Design review of the part built by this model. Coordinates are the model's own, in mm. A direction names the side the tool comes from. Give positions to 0.01 mm unless a question says otherwise; leave off trailing zeros. Order: outer loops, then holes, each group sorted by start corner. A loop starts at its lowest first (then second) coordinate and runs counter-clockwise, first axis right, second up. Notation, with made-up numbers: (36.25, 20) -> (45.25, 20) arc R20 ccw to (45.25, 30) -> close; hole circle Ø2 at (25, 15). An arc over 180 degrees is marked (long way). Return JSON: item names as keys, results as strings.
```python
from build123d import *

# Parameters (mm, degrees)
SKETCH1_R                                            = 60
SKETCH1_R_2                                          = 45
SKETCH1_R_3                                          = 40
BOSS_EXTRUDE3_DEPTH                                  = 10
SKETCH4_R                                            = 60
SKETCH4_R_2                                          = 50
BOSS_EXTRUDE4_DEPTH                                  = 6
SKETCH5_R                                            = 45
SKETCH5_R_2                                          = 42.5
BOSS_EXTRUDE5_DEPTH                                  = 8
FILLET1_R                                            = 2
SKETCH6_R                                            = 52.5
SKETCH6_R_2                                          = 42.5
CUT_EXTRUDE2_DEPTH                                   = 2
BOSS_EXTRUDE6_DEPTH                                  = 30
BOSS_EXTRUDE7_REACH                                  = 311.38
SKETCH8_R                                            = 20.5
SKETCH9_R                                            = 15
BOSS_EXTRUDE8_DEPTH                                  = 20
CUT_EXTRUDE3_DEPTH                                   = 250.99199991
CBORE_FOR_M3_HEXAGON_HEAD_BOLTS_FULL_THR_D           = 3.4
CBORE_FOR_M3_HEXAGON_HEAD_BOLTS_FULL_THR_CBORE_D     = 7
CBORE_FOR_M3_HEXAGON_HEAD_BOLTS_FULL_THR_CBORE_DEPTH = 2
CBORE_FOR_M3_HEXAGON_HEAD_BOLTS_FULL_2_D             = 3.4
CBORE_FOR_M3_HEXAGON_HEAD_BOLTS_FULL_2_CBORE_D       = 7
CBORE_FOR_M3_HEXAGON_HEAD_BOLTS_FULL_2_CBORE_DEPTH   = 2
SKETCH17_R                                           = 2.05
CUT_EXTRUDE4_DEPTH                                   = 15
SKETCH18_R                                           = 2.05
CUT_EXTRUDE5_DEPTH                                   = 15
SKETCH19_R                                           = 6
CUT_EXTRUDE6_DEPTH                                   = 2.5
SKETCH20_R                                           = 6
CUT_EXTRUDE7_DEPTH                                   = 2.5


with BuildPart() as part:
    # Sketch1 → Boss-Extrude3 (new body)
    # profile 1 of 3: a face of its own
    with BuildSketch(Plane(origin=(0, 0, 0), x_dir=(0, 0, -1), z_dir=(1, 0, 0))):
        Circle(SKETCH1_R)
        Circle(SKETCH1_R_2, mode=Mode.SUBTRACT)
    # profile 2 of 3: a face of its own
    with BuildSketch(Plane(origin=(0, 0, 0), x_dir=(0, 0, -1), z_dir=(1, 0, 0))):
        with BuildLine():
            ThreePointArc((-23.076923077, 55.384615385), (-60.776772972, 43.883864862), (-100, 40))
            Line((-100, 40), (-200, 40))
            ThreePointArc((-200, 40), (-171.715728753, 28.284271247), (-160, 0))
            ThreePointArc((-160, 0), (-171.715728753, -28.284271247), (-200, -40))
            Line((-200, -40), (-100, -40))
            ThreePointArc((-100, -40), (-60.776772972, -43.883864862), (-23.076923077, -55.384615385))
            ThreePointArc((-23.076923077, -55.384615385), (-60, 0), (-23.076923077, 55.384615385))
        make_face()
    # profile 3 of 3: a face of its own
    with BuildSketch(Plane(origin=(0, 0, 0), x_dir=(0, 0, -1), z_dir=(1, 0, 0))):
        with Locations((-200, 0)):
            Circle(SKETCH1_R_3)
    extrude(amount=BOSS_EXTRUDE3_DEPTH)

    # Sketch4 → Boss-Extrude4 (add)
    with BuildSketch(Plane(origin=(10, 0, 0), x_dir=(0, 0, -1), z_dir=(1, 0, 0))):
        with Locations(Location((0, 0, 0), (0, 0, 112.619864948))):
            Circle(SKETCH4_R)
        Circle(SKETCH4_R_2, mode=Mode.SUBTRACT)
    extrude(amount=BOSS_EXTRUDE4_DEPTH)

    # Sketch5 → Boss-Extrude5 (add)
    with BuildSketch(Plane.ZY):
        with Locations(Location((0, 0, 0), (0, 0, 180))):
            Circle(SKETCH5_R)
        Circle(SKETCH5_R_2, mode=Mode.SUBTRACT)
    extrude(amount=-BOSS_EXTRUDE5_DEPTH)

    # Fillet1
    fillet1_edges = [part.edges().sort_by_distance(p)[0] for p in [
        (8, 0, 45),
    ]]
    fillet(fillet1_edges, radius=FILLET1_R - 0.0001)  # a hair under: the kernel refuses the full size

    # Sketch6 → Cut-Extrude2 (cut)
    with BuildSketch(Plane.ZY):
        Circle(SKETCH6_R)
        Circle(SKETCH6_R_2, mode=Mode.SUBTRACT)
    extrude(amount=-CUT_EXTRUDE2_DEPTH, mode=Mode.SUBTRACT)

    # Sketch7 → Boss-Extrude6 (add)
    with BuildSketch(Plane(origin=(16, 0, 0), x_dir=(0, 0, -1), z_dir=(1, 0, 0))):
        with BuildLine():
            ThreePointArc((60, 0), (42.426406871, 42.426406871), (0, 60))
            Line((0, 60), (0, 52))
            ThreePointArc((0, 52), (52, 0), (0, -52))
            Line((0, -52), (0, -60))
            ThreePointArc((0, -60), (42.426406871, -42.426406871), (60, 0))
        make_face()
    extrude(amount=BOSS_EXTRUDE6_DEPTH)

    # Sketch8 → Boss-Extrude7 (add, up to next)
    with BuildSketch(Plane(origin=(0, 0, -60), x_dir=(-1, 0, 0), z_dir=(0, 0, -1)), mode=Mode.PRIVATE) as boss_extrude7_sk1:
        with Locations((-25.5, 0)):
            Circle(SKETCH8_R)
    boss_extrude7_tool1 = extrude(boss_extrude7_sk1.sketch, amount=-BOSS_EXTRUDE7_REACH, mode=Mode.PRIVATE) - part.part
    add(boss_extrude7_tool1.solids().sort_by_distance((25.5, 0, -60))[0])
    add(boss_extrude7_tool1.solids().sort_by_distance((25.5, 0, -60))[1])

    # Sketch9 → Boss-Extrude8 (add)
    with BuildSketch(Plane(origin=(0, 0, -60), x_dir=(-1, 0, 0), z_dir=(0, 0, -1))):
        with Locations((-25.5, 0)):
            Circle(SKETCH9_R)
    extrude(amount=BOSS_EXTRUDE8_DEPTH)

    # Sketch12 → Cut-Extrude3 (cut, through all)
    with BuildSketch(Plane(origin=(10, 0, 0), x_dir=(0, 0, -1), z_dir=(1, 0, 0))):
        with BuildLine():
            Line((-200, 30), (-200, 40))
            ThreePointArc((-200, 40), (-240, 0), (-200, -40))
            Line((-200, -40), (-200, -30))
            ThreePointArc((-200, -30), (-230, 0), (-200, 30))
        make_face()
    extrude(amount=-CUT_EXTRUDE3_DEPTH, mode=Mode.SUBTRACT)

    # CBORE for M3 Hexagon head bolts-Full thread-grades AB2 (through all)
    with Locations(Plane(origin=(41, 54.543560573, -25), x_dir=(0, 0.416666666667, 0.909059342886), z_dir=(0, 0.909059342886, -0.416666666667))):
        with Locations((0, 0)):
            CounterBoreHole(CBORE_FOR_M3_HEXAGON_HEAD_BOLTS_FULL_THR_D / 2, CBORE_FOR_M3_HEXAGON_HEAD_BOLTS_FULL_THR_CBORE_D / 2, CBORE_FOR_M3_HEXAGON_HEAD_BOLTS_FULL_THR_CBORE_DEPTH)

    # CBORE for M3 Hexagon head bolts-Full 2 (through all)
    with Locations(Plane(origin=(41, -54.543560573, -25), x_dir=(0, 0.416667072006, -0.909059157099), z_dir=(0, -0.909059157099, -0.416667072006))):
        with Locations((0, 0)):
            CounterBoreHole(CBORE_FOR_M3_HEXAGON_HEAD_BOLTS_FULL_2_D / 2, CBORE_FOR_M3_HEXAGON_HEAD_BOLTS_FULL_2_CBORE_D / 2, CBORE_FOR_M3_HEXAGON_HEAD_BOLTS_FULL_2_CBORE_DEPTH)

    # Sketch17 → Cut-Extrude4 (cut)
    with BuildSketch(Plane(origin=(0, -119.511505722, 69), x_dir=(-1, 0, 0), z_dir=(0, -0.8660254037844414, 0.49999999999999517))):
        with Locations(Location((-5, -173.205080757, 0), (0, 0, 90))):
            Circle(SKETCH17_R)
    extrude(amount=-CUT_EXTRUDE4_DEPTH, mode=Mode.SUBTRACT)

    # Sketch18 → Cut-Extrude5 (cut)
    with BuildSketch(Plane(origin=(0, 119.511505722, 69), x_dir=(1, 0, 0), z_dir=(0, 0.8660254037844414, 0.49999999999999517))):
        with Locations(Location((5, -173.205080757, 0), (0, 0, 270))):
            Circle(SKETCH18_R)
    extrude(amount=-CUT_EXTRUDE5_DEPTH, mode=Mode.SUBTRACT)

    # Sketch19 → Cut-Extrude6 (cut)
    with BuildSketch(Plane(origin=(10, 0, 0), x_dir=(0, 0, -1), z_dir=(1, 0, 0))):
        with Locations((-200, 0)):
            Circle(SKETCH19_R)
    extrude(amount=-CUT_EXTRUDE6_DEPTH, mode=Mode.SUBTRACT)

    # Sketch20 → Cut-Extrude7 (cut)
    with BuildSketch(Plane(origin=(10, 0, 0), x_dir=(0, 0, -1), z_dir=(1, 0, 0))):
        with Locations((-80, -25)):
            Circle(SKETCH20_R)
        with Locations((-80, 25)):
            Circle(SKETCH20_R)
    extrude(amount=-CUT_EXTRUDE7_DEPTH, mode=Mode.SUBTRACT)


solid = part.part
```
Item 1: Machinability: for faces 1 (the face through (7.5, 25, 80)), 2 (the face through (5, -35, 200)), 3 (the face through (31, -56, 0)), which of the approach directions +Z, -Z, +X, -X, +Y, -Y give a long, thin tool a straight path to every point of the face, cutting with its end or side? Answer none if there is none.
Result set:
{"face 1": "+X", "face 2": "+Z, +X, -X, -Y", "face 3": "+Z, +X, +Y, -Y"}
Item 2: Mouldability with a two-part tool opening along X and no side actions: class faces 4 (the face through (4.215, -23.94, 211.635)), 5 (the face through (5, 40, 149)), 6 (the face through (10, 19, 41)) as released by +X, released by -X, zero draft, split by the parting line, or undercut.
Result set:
{"face 4": "undercut", "face 5": "zero draft", "face 6": "released by +X"}
Item 3: For pin 1 (5 mm diameter, centred on x = 35.5, y = 24.5, fed in from -Z); pin 2 (14 mm diameter, centred on y = -25, z = 80, fed in from +X); pin 3 (2 mm diameter, centred on x = 22, z = -29, fed in from +Y), all flat-tipped, find the tip position at first contact; note any pin that passes through.
Result set:
{"pin 1": "stops at z = -55.82", "pin 2": "stops at x = 10", "pin 3": "stops at y = 53.07"}
Item 4: Add section A-A (x = 25.5). Give the boundary of the cut face in (y, z), plus the area to 3 significant figures.
Result set:
{"outline": "(-60, 0) arc R60 ccw to (-20.5, -56.39) -> (-20.5, -60) -> (-15, -60) -> (-15, -80) -> (15, -80) -> (15, -60) -> (20.5, -60) -> (20.5, -56.39) arc R60 ccw to (60, 0) -> (52, 0) arc R52 cw to (-52, 0) -> close", "area": "2,060 mm^2"}
Item 5: Wall thickness on L1, parallel to Y at x = 27, z = -2; L2, parallel to X at y = -6, z = 203.5; L3, parallel to Y at x = 13, z = 0: over which ranges is each line inside the solid? List them lowest first. Write a range as [from, to].
Result set:
{"L1": "y = [-59.97, -51.96], [51.96, 59.97]", "L2": "x = [0, 10]", "L3": "y = [-60, -50], [50, 60]"}
Item 6: Add section B-B (z = 104). Give the boundary of the cut face in (x, y).
Result set:
{"outline": "(0, -40) -> (10, -40) -> (10, 40) -> (0, 40) -> close"}
